from build123d import *

# Parameters (mm, degrees)
F0_W     = 55
F0_H     = 11
F0_H_2   = 5
F1_DEPTH = 8
F0_R     = 1.75
F2_DEPTH = 4
F3_DEPTH = 3.5


with BuildPart() as f1:
    # F0 (on Top) → F1 (new body)
    with BuildSketch(Plane.XY):
        with Locations((0, -2.5)):
            Rectangle(F0_W, F0_H)
        Polygon((-16.824574, -2), (-18.412287, -4.75), (-21.587713, -4.75), (-23.175426, -2), (-21.587713, 0.75), (-18.412287, 0.75), align=None, mode=Mode.SUBTRACT)
        Polygon((0, 1.175426), (2.75, -0.412287), (2.75, -3.587713), (0, -5.175426), (-2.75, -3.587713), (-2.75, -0.412287), align=None, mode=Mode.SUBTRACT)
        Polygon((18.412287, -4.75), (16.824574, -2), (18.412287, 0.75), (21.587713, 0.75), (23.175426, -2), (21.587713, -4.75), align=None, mode=Mode.SUBTRACT)
        with Locations((0, 5.5)):
            Rectangle(F0_W, F0_H_2)
        Polygon((-27.5, 8), (27.5, 8), (7.497111, 27.834252), (0, 15.674993), (-7.823137, 27.510974), align=None)
        with BuildLine():
            Line((7.497111, 27.834252), (27.5, 8))
            ThreePointArc((27.5, 8), (30.409967, 15.459144), (37.60235, 18.97715))
            ThreePointArc((37.60235, 18.97715), (-0.876943, 35.275336), (-39.356235, 18.97715))
            ThreePointArc((-39.356235, 18.97715), (-31.029945, 16.078802), (-27.5, 8))
            Line((-27.5, 8), (-7.823137, 27.510974))
            Line((-7.823137, 27.510974), (-0.934656, 34.341381))
            Line((-0.934656, 34.341381), (0.934656, 34.341381))
            Line((0.934656, 34.341381), (7.497111, 27.834252))
        make_face()
    extrude(amount=F1_DEPTH)

    # F0 (on Top) → F2 (join)
    with BuildSketch(Plane.XY):
        Polygon((-21.587713, -4.75), (-18.412287, -4.75), (-16.824574, -2), (-18.412287, 0.75), (-21.587713, 0.75), (-23.175426, -2), align=None)
        with Locations((-20, -2)):
            Circle(F0_R, mode=Mode.SUBTRACT)
        Polygon((2.75, -3.587713), (2.75, -0.412287), (0, 1.175426), (-2.75, -0.412287), (-2.75, -3.587713), (0, -5.175426), align=None)
        with Locations((0, -2)):
            Circle(F0_R, mode=Mode.SUBTRACT)
        Polygon((18.412287, 0.75), (16.824574, -2), (18.412287, -4.75), (21.587713, -4.75), (23.175426, -2), (21.587713, 0.75), align=None)
        with Locations((20, -2)):
            Circle(F0_R, mode=Mode.SUBTRACT)
    extrude(amount=F2_DEPTH)

    # F0 (on Top) → F3 (join)
    with BuildSketch(Plane.XY):
        with Locations((0, 5.5)):
            Rectangle(F0_W, F0_H_2)
    extrude(amount=-F3_DEPTH)


solid = f1.part
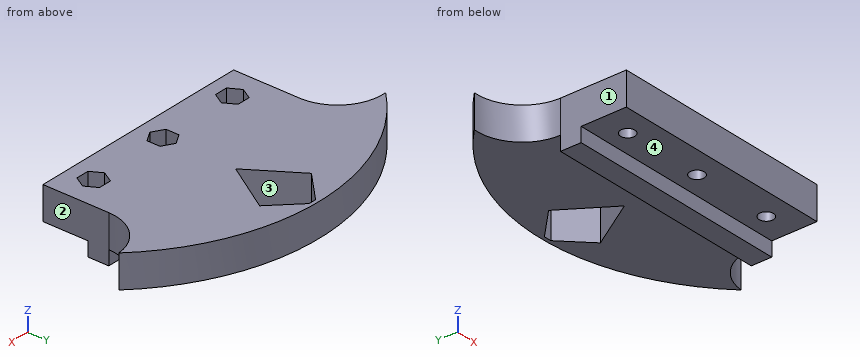
Read the model definition and answer for the solid it produces. Units are mm, in the model's axes. Face numbers are marked on the shaded views. A direction names the side the tool comes from. Give positions to 0.01 mm unless a question says otherwise; leave off trailing zeros. Write each loop counter-clockwise with the first axis right and the second up, starting at its lowest first coordinate (ties: lowest second). Pieces come first, ordered by that corner, then holes. Notation, with made-up numbers: (9.25, -36) - (21.25, -36) arc R8 cw to (21.25, -22) - close; hole circle Ø6 at (28, 62.25). An arc over 180 degrees is marked (long way). Use CSV: the item, a comma, the result in double quotes. Start each with the question number.
Item 1: Consider line 1 (X direction, y = -2.5, z = 5.25); line 2 (Y direction, x = -1.5, z = 2.5); line 3 (Y direction, x = 22.5, z = -1.75). Determine where each line is inside the solid, lowest interval first.
Item 2: The part is cut by section A-A, the plane z = 5. Count the separate pieces of the cut face and the enclosed holes in it, and give its area (3 significant figures).
Item 3: The part is cut by section D-D, the plane z = 1.75. Give the vertices of the cut face in (x, y) (3 decimals).
Item 4: The part is cut by section C-C, the plane x = -20. Give the vertices of the cut face in (y, z).
Item 5: Flat-ended cylindrical pins translate along their axes: P1, Ø3.5, axis at x = -7.5, y = -3.5, coming from the -Z side; P2, Ø3, axis at x = 2, z = -2.5, coming from the -Y side; P3, Ø2, axis at x = 20, y = -2, coming from the +Z side; P4, Ø1, axis at y = 27.5, z = 6, coming from the +X side. Find the tip coordinate at first contact, or state that the pin passes through.
Item 6: The part is cut by section B-B, the plane y = 32. Give the vertices of the cut face in (x, z), and give its area (3 significant figures).
Item 7: For the marked faces 1, 2, 3 and 4, determine the directions among +Z, -Z, +X, -X, +Y, -Y from which every point of the face is accessible in a straight line to the end or side of a thin tool.
Taken from the geometry:
1,line 1,"-27.5 to -22.89, -17.11 to -2.75, 2.75 to 17.11, 22.89 to 27.5"
1,line 2,"-8 to -2.9, -1.1 to 17.94, 33.78 to 35.27"
1,line 3,"3 to 8"
2,separate pieces,"1"
2,enclosed holes,"4"
2,area,"2,170 mm2"
3,outline,"(-39.356, 18.977) arc R11.01 cw to (-27.5, 8) - (-27.5, -8) - (27.5, -8) - (27.5, 8) arc R11.015 cw to (37.602, 18.977) arc R53.573 ccw to start; hole circle Ø3.5 at (-20, -2); hole (-7.823, 27.511) - (0, 15.675) - (7.497, 27.834) - (0.935, 34.341) - (-0.935, 34.341) - close; hole circle Ø3.5 at (0, -2); hole circle Ø3.5 at (20, -2)"
4,outline,"(-8, 0) - (-3.75, 0) - (-3.75, 4) - (-4.75, 4) - (-4.75, 8) - (-8, 8) - close; (-0.25, 0) - (3, 0) - (3, -3.5) - (8, -3.5) - (8, 0) - (31.75, 0) - (31.75, 8) - (0.75, 8) - (0.75, 4) - (-0.25, 4) - close"
5,P1,"z = 0"
5,P2,"y = 3"
5,P3,"through"
5,P4,"x = 27.73"
6,outline,"(-19.32, 0) - (-3.3, 0) - (-3.3, 8) - (-19.32, 8) - close; (3.3, 0) - (17.57, 0) - (17.57, 8) - (3.3, 8) - close"
6,area,"242 mm2"
7,face 1,"+Z, -Z, -X, -Y"
7,face 2,"+Z, -Z, +X, -Y"
7,face 3,"+Z, -Z"
7,face 4,"-Z, +X, -X, -Y"
